Geometry check sheet. Reference: the model listing, model coordinates, mm. A direction names the side the tool comes from. Round coordinates to 2 decimals unless told otherwise and drop trailing zeros. Write each loop counter-clockwise with the first axis right and the second up, starting at its lowest first coordinate (ties: lowest second). Pieces come first, ordered by that corner, then holes. Notation, with made-up numbers: (-38.75, 27.5) -> (-27.75, 27.5) arc R21 cw to (-27.75, 51.5) -> close; hole circle Ø9 at (22, 3). An arc over 180 degrees is marked (long way). Use a Markdown table: item, result.
```python
from build123d import *

# Parameters (mm, degrees)
F0_W     = 5.08
F0_H     = 5.08
F0_W_2   = 15.24
F0_W_3   = 50.8
F0_H_2   = 172.72
F1_DEPTH = 5.08
F2_W     = 5.08
F2_H     = 5.08
F3_DEPTH = 50.8
F4_W     = 5.08
F4_H     = 5.08
F5_DEPTH = 15.24
F6_W     = 5.08
F6_H     = 5.08
F7_DEPTH = 15.24


with BuildPart() as f1:
    # F0 (on Top) → F1 (new body)
    with BuildSketch(Plane.XY):
        with Locations((-74.2818623495, 91.6018860722)):
            Rectangle(F0_W, F0_H)
        with Locations((-84.4418623495, 91.6018860722)):
            Rectangle(F0_W_2, F0_H)
        with Locations((-46.3418623495, 91.6018860722)):
            Rectangle(F0_W_3, F0_H)
        with Locations((-74.2818623495, 2.7018860722)):
            Rectangle(F0_W, F0_H_2)
        with Locations((-18.4018623495, 91.6018860722)):
            Rectangle(F0_W, F0_H)
        with Locations((-74.2818623495, -86.1981139278)):
            Rectangle(F0_W, F0_H)
        with Locations((-84.4418623495, -86.1981139278)):
            Rectangle(F0_W_2, F0_H)
        with Locations((-46.3418623495, -86.1981139278)):
            Rectangle(F0_W_3, F0_H)
        with Locations((-18.4018623495, 2.7018860722)):
            Rectangle(F0_W, F0_H_2)
        with Locations((-8.2418623495, 91.6018860722)):
            Rectangle(F0_W_2, F0_H)
        with Locations((-18.4018623495, -86.1981139278)):
            Rectangle(F0_W, F0_H)
        with Locations((-8.2418623495, -86.1981139278)):
            Rectangle(F0_W_2, F0_H)
    extrude(amount=F1_DEPTH)

    # F2 (on face) → F3 (join)
    with BuildSketch(Plane.YZ.offset(-71.7418623495)):
        with Locations((-65.8781139278, 2.54)):
            Rectangle(F2_W, F2_H)
    extrude(amount=F3_DEPTH)

    # F4 (on face) → F5 (join)
    with BuildSketch(Plane.YZ.offset(-15.8618623495)):
        with Locations((-65.8781139278, 2.54)):
            Rectangle(F4_W, F4_H)
    extrude(amount=F5_DEPTH)

    # F6 (on face) → F7 (join)
    with BuildSketch(Plane(origin=(-76.8218623495, 0, 0), x_dir=(0, -1, 0), z_dir=(-1, 0, 0))):
        with Locations((65.8781139278, 2.54)):
            Rectangle(F6_W, F6_H)
    extrude(amount=F7_DEPTH)


solid = f1.part
```
(1) Gauge pin test, flat ends, axial feed: pin 1 Ø2.5 at (y, z) = (-72.5, 3.5) entering from +X; pin 2 Ø1.5 at (y, z) = (-79, 3) entering from -X; pin 3 Ø8 at (x, y) = (-65.5, 56.5) entering from +Z. Record the tip position at first contact, or that the pin passes through.
A:
| item | result |
|---|---|
| pin 1 | stops at x = -15.86 |
| pin 2 | stops at x = -76.82 |
| pin 3 | passes through |
(2) Section check B-B on x = -69. Record the cut outline in (y, z), plus the area to 3 significant figures.
A:
| item | result |
|---|---|
| outline | (-88.74, 0) -> (-83.66, 0) -> (-83.66, 5.08) -> (-88.74, 5.08) -> close; (-68.42, 0) -> (-63.34, 0) -> (-63.34, 5.08) -> (-68.42, 5.08) -> close; (89.06, 0) -> (94.14, 0) -> (94.14, 5.08) -> (89.06, 5.08) -> close |
| area | 77.4 mm2 |
(3) Thickness scan on line 1 (Y direction, x = -30.5, z = 0.2); line 2 (X direction, y = 42, z = 4.55). Record the ranges inside material, lowest first.
A:
| item | result |
|---|---|
| line 1 | y = -88.74 to -83.66, -68.42 to -63.34, 89.06 to 94.14 |
| line 2 | x = -76.82 to -71.74, -20.94 to -15.86 |
(4) Access from +Z, -Z, +X, -X, +Y, -Y to the whole of each face (thin tool, end or side, straight path). Record for faces 4 (the face through (-92.062, -86, 3)), 5 (the face through (-85, -83.658, 3)), 6 (the face through (-0.622, -86, 3)), 7 (the face through (-47, -63.338, 3)), 8 (the face through (-8, -68.418, 3)).
A:
| item | result |
|---|---|
| face 4 | +Z, -Z, -X, +Y, -Y |
| face 5 | +Z, -Z, -X |
| face 6 | +Z, -Z, +X, +Y, -Y |
| face 7 | +Z, -Z |
| face 8 | +Z, -Z, +X |
(5) Release check for a two-part mould opening along Y. For faces 1 (the face through (-46, 94.142, 3)), 2 (the face through (-20.942, -76, 3)), 3 (the face through (-92.062, -66, 3)) record: +Y half, -Y half, draft (parallel to the pull), parting line (faces both ways), or undercut.
A:
| item | result |
|---|---|
| face 1 | +Y half |
| face 2 | undercut |
| face 3 | draft |
(6) Section check C-C on z = 3.25. Record the cut outline in (x, y).
A:
| item | result |
|---|---|
| outline | (-92.06, -88.74) -> (-0.62, -88.74) -> (-0.62, -83.66) -> (-15.86, -83.66) -> (-15.86, -68.42) -> (-0.62, -68.42) -> (-0.62, -63.34) -> (-15.86, -63.34) -> (-15.86, 89.06) -> (-0.62, 89.06) -> (-0.62, 94.14) -> (-92.06, 94.14) -> (-92.06, 89.06) -> (-76.82, 89.06) -> (-76.82, -63.34) -> (-92.06, -63.34) -> (-92.06, -68.42) -> (-76.82, -68.42) -> (-76.82, -83.66) -> (-92.06, -83.66) -> close; hole (-71.74, -83.66) -> (-20.94, -83.66) -> (-20.94, -68.42) -> (-71.74, -68.42) -> close; hole (-71.74, -63.34) -> (-20.94, -63.34) -> (-20.94, 89.06) -> (-71.74, 89.06) -> close |
(7) Section check A-A on y = -53. Record the cut outline in (x, z), plus the area to 3 significant figures.
A:
| item | result |
|---|---|
| outline | (-76.82, 0) -> (-71.74, 0) -> (-71.74, 5.08) -> (-76.82, 5.08) -> close; (-20.94, 0) -> (-15.86, 0) -> (-15.86, 5.08) -> (-20.94, 5.08) -> close |
| area | 51.6 mm2 |
